Can you work these out from the model? Positions are in its coordinate system, mm. A direction names the side the tool comes from. Give positions to 0.01 mm unless a question says otherwise; leave off trailing zeros. Loops run counter-clockwise (first coordinate to the right, second up) from the corner with the lowest first, then second, coordinate; pieces in that order, holes last. Notation, with made-up numbers: (-40, -40) - (-15, -40) arc R24 ccw to (-15, -6) - close; hole circle Ø4 at (-33, -38.5). An arc over 180 degrees is marked (long way). Write item = value, one per line.
from build123d import *

# Parameters (mm, degrees)
BOSS_EXTRUDE1_DEPTH = 1
FILLET1_R           = 5
FILLET2_R           = 0.5


with BuildPart() as part:
    # Sketch1 → Boss-Extrude1 (new body)
    with BuildSketch(Plane(origin=(0, 0, 0), x_dir=(1, 0, 0), z_dir=(0, 1, 0))):
        Polygon((-25, -18.9), (25, -18.9), (25, -14.1), (22.96, -14.1), (22.96, 13.9), (25, 13.9), (25, 18.9), (-25, 18.9), (-25, 13.9), (-23, 13.9), (-23, -14.1), (-25, -14.1), align=None)
        with BuildLine():
            Line((-18.351, 15.911365238), (17.970976359, 15.911365238))
            Line((17.970976359, 15.911365238), (17.971, 14))
            Line((17.971, 14), (19.96, 14))
            ThreePointArc((19.96, 14), (20.667106781, 13.707106781), (20.96, 13))
            Line((20.96, 13), (20.96, -13))
            ThreePointArc((20.96, -13), (20.667106781, -13.707106781), (19.96, -14))
            Line((19.96, -14), (17.971, -14))
            Line((17.971, -14), (17.971, -15.911365238))
            Line((17.971, -15.911365238), (-18.351, -15.911365238))
            Line((-18.351, -15.911365238), (-18.351, -14))
            Line((-18.351, -14), (-20, -14))
            ThreePointArc((-20, -14), (-20.711257423, -13.702939741), (-21, -12.988265238))
            Line((-21, -12.988265238), (-21, 12.988265238))
            ThreePointArc((-21, 12.988265238), (-20.711254501, 13.702936852), (-20, 14))
            Line((-20, 14), (-18.351, 14))
            Line((-18.351, 14), (-18.351, 15.911365238))
        make_face(mode=Mode.SUBTRACT)
    extrude(amount=BOSS_EXTRUDE1_DEPTH)

    # Fillet1
    # the kernel refuses this fillet: 5 mm, written as the material it takes off along each edge
    with BuildSketch(Plane(origin=(25, -12.489995997, 18.9), x_dir=(-1, 0, 0), z_dir=(0, 1, 0))) as fillet1_piece_1:
        with BuildLine():
            CenterArc((4.995998399, -5), FILLET1_R, 90, 87.707557224)
            Line((0, -4.8), (-0.099919968, -4.796))
            ThreePointArc((-0.099919968, -4.796), (-0.1, -2.4), (-0.1, 0))
            Line((-0.1, 0), (0, 0.1))
            Line((0, 0.1), (4.995998399, 0.1))
            Line((4.995998399, 0.1), (4.995998399, 0))
        make_face()
    extrude(amount=25.979991994, mode=Mode.SUBTRACT)
    with BuildSketch(Plane(origin=(-25, -12.489995997, 18.9), x_dir=(1, 0, 0), z_dir=(0, 1, 0))) as fillet1_piece_2:
        with BuildLine():
            CenterArc((4.995998399, 5), FILLET1_R, 182.292442776, 87.707557224)
            Line((0, 4.8), (-0.099919968, 4.796))
            ThreePointArc((-0.099919968, 4.796), (-0.1, 2.4), (-0.1, 0))
            Line((-0.1, 0), (0, -0.1))
            Line((0, -0.1), (4.995998399, -0.1))
            Line((4.995998399, -0.1), (4.995998399, 0))
        make_face()
    extrude(amount=25.979991994, mode=Mode.SUBTRACT)
    with BuildSketch(Plane(origin=(-25, -12.5, -18.9), x_dir=(1, 0, 0), z_dir=(0, 1, 0)), Plane(origin=(25, -12.5, -18.9), x_dir=(0, 0, 1), z_dir=(0, 1, 0))) as fillet1_piece_3:
        with BuildLine():
            CenterArc((FILLET1_R, -FILLET1_R), FILLET1_R, 90, 90)
            Line((0, -FILLET1_R), (-FILLET1_R * 0.02, -FILLET1_R))
            Line((-FILLET1_R * 0.02, -FILLET1_R), (-FILLET1_R * 0.02, FILLET1_R * 0.02))
            Line((-FILLET1_R * 0.02, FILLET1_R * 0.02), (FILLET1_R, FILLET1_R * 0.02))
            Line((FILLET1_R, FILLET1_R * 0.02), (FILLET1_R, 0))
        make_face()
    extrude(amount=26, mode=Mode.SUBTRACT)

    # Fillet2
    fillet2_edges = [part.edges().sort_by_distance(p)[0] for p in [
        (-24, 1, -13.9),
        (-23, 1, 0.1),
        (-24, 1, 14.1),
        (23.98, 1, 14.1),
        (22.96, 1, 0.1),
        (23.98, 1, -13.9),
        (-19.1755, 1, -14),
        (-20.711254501, 1, -13.702936852),
        (-21, 1, 0),
        (-20.711257423, 1, 13.702939741),
        (-19.1755, 1, 14),
        (18.9655, 1, 14),
        (20.667106781, 1, 13.707106781),
        (20.96, 1, 0),
        (20.667106781, 1, -13.707106781),
        (18.9655, 1, -14),
        (0, 1, -18.9),
        (0, 1, 18.9),
        (-23.468103216, 1, 17.505551275),
        (23.468103216, 1, 17.505551275),
        (23.535533906, 1, -17.435533906),
        (-23.535533906, 1, -17.435533906),
    ]]
    fillet(fillet2_edges, radius=FILLET2_R)


solid = part.part
Q1. Imagine slicing it at C-C, the plane y = 0.2. Write out the boundary of the cut face in (x, z), then the cut area to 3 significant figures.
Output:
outline = (-25, -13.9) arc R5 ccw to (-20, -18.9) - (20, -18.9) arc R5 ccw to (25, -13.9) - (22.96, -13.9) - (22.96, 14.1) - (25, 14.1) arc R5 ccw to (20, 18.9) - (-20, 18.9) arc R5 ccw to (-25, 14.1) - (-23, 14.1) - (-23, -13.9) - close; hole (-21, -12.99) arc R1 ccw to (-20, -14) - (-18.35, -14) - (-18.35, -15.91) - (17.97, -15.91) - (17.97, -14) - (19.96, -14) arc R1 ccw to (20.96, -13) - (20.96, 13) arc R1 ccw to (19.96, 14) - (17.97, 14) - (17.97, 15.91) - (-18.35, 15.91) - (-18.35, 14) - (-20, 14) arc R1 ccw to (-21, 12.99) - close
area = 443 mm2
Q2. I need wall thicknesses on L1, parallel to X at y = 0.55, z = -11; L2, parallel to Z at x = -12, y = 0.2; L3, parallel to X at y = 0.75, z = -5. Which ranges of each line are inside material? Lowest first, please.
Output:
L1 = -23 to -21, 20.96 to 22.96
L2 = -18.9 to -15.91, 15.91 to 18.9
L3 = -22.93 to -21.07, 21.03 to 22.89
Q3. Imagine slicing it at A-A, the plane z = 7. Write out the boundary of the cut face in (x, y).
Output:
outline = (-23, 0) - (-21, 0) - (-21, 0.5) arc R0.5 ccw to (-21.5, 1) - (-22.5, 1) arc R0.5 ccw to (-23, 0.5) - close; (20.96, 0) - (22.96, 0) - (22.96, 0.5) arc R0.5 ccw to (22.46, 1) - (21.46, 1) arc R0.5 ccw to (20.96, 0.5) - close
Q4. We'd pull the mould along Z, two halves only. Please class faces 3 (the cylindrical face through (-23.507, 0.246, 17.468)), 4 (the flat face through (-18.351, 0.5, 15)), 5 (the flat face through (-0.1, 1, 16.3)), 6 (the cylindrical face through (20.659, 0.247, -13.715)): released by +Z, released by -Z, zero draft, split by the parting line, or undercut.
Output:
face_3 = released by +Z
face_4 = undercut
face_5 = zero draft
face_6 = undercut
Q5. Imagine slicing it at B-B, the plane x = 12. Write out the boundary of the cut face in (y, z).
Output:
outline = (0, -18.9) - (0.5, -18.9) arc R0.5 ccw to (1, -18.4) - (1, -15.91) - (0, -15.91) - close; (0, 15.91) - (1, 15.91) - (1, 18.4) arc R0.5 ccw to (0.5, 18.9) - (0, 18.9) - close
Q6. Which directions (+Z, -Z, +X, -X, +Y, -Y) give clear straight access to the entire face, cutting with the end or side of a thin tool? Please do faces 1 (the flat face through (0, 0, 17)), 2 (the cylindrical face through (20.675, 0.247, 13.699)).
Output:
face_1 = +Z, -Z, +X, -X, -Y
face_2 = +Y, -Y
Q7. For pin 1 (0.6 mm diameter, centred on y = 0.5, z = -5.5, fed in from +X); pin 2 (0.6 mm diameter, centred on x = -24, y = 0, fed in from +Z); pin 3 (0.6 mm diameter, centred on x = 24, y = 0.5, fed in from -Z); pin 4 (2 mm diameter, centred on x = -10, z = -13.5, fed in from -Y), each with a flat end and sliding along its axis, tell me the tip position at first contact or that it passes through.
Output:
pin_1 = 22.96
pin_2 = 17.27
pin_3 = -17.26
pin_4 = through
